Model file for the job. Use its own axes, mm. A direction names the side the tool comes from. Round coordinates to 2 decimals unless told otherwise and drop trailing zeros. Order: outer loops, then holes, each group sorted by start corner. A loop starts at its lowest first (then second) coordinate and runs counter-clockwise, first axis right, second up. Notation, with made-up numbers: M 23.25,27 L 29.25,27 A22 ccw 29.25,48 Z; hole C -28,-19.5 d5. An arc over 180 degrees is marked long. Return JSON: item names as keys, results as strings. Group by question number.
Item 1: Which spindle directions (+Z, -Z, +X, -X, +Y, -Y) get a long thin tool onto all of the face, cutting with end or side? Do faces 5 (the face through (18, -1, 12.5)), 6 (the face through (34, -2, 6)), 7 (the face through (17, -3.2, 7)), 8 (the face through (19, -2, 11.7)), 9 (the face through (4, -2, 6)). Say none if no direction does.
Item 2: Slice it at D-D on z = 5.75. Write the cut outline in (x, y).
Item 3: Pin check, flat tips, straight feed: pin 1 Ø1.3 at (x, y) = (20, -3) entering from +Z; pin 2 Ø0.5 at (y, z) = (-2.5, 7.5) entering from +X. Stop position of each tip, or through.
Item 4: Pull direction Z, two halves, no side cores. Call faces 1 (the face through (19, -3.3, 3)), 2 (the face through (19, -2, 0.2)), 3 (the face through (1.215, -0.838, 5.317)), 4 (the face through (0.948, -0.838, 7.917)): pulls with the +Z half, pulls with the -Z half, needs draft (parallel to the pull), parting line crosses it, or undercut.
Item 5: Slice it at B-B on z = 7.52. Write the cut outline in (x, y).
Item 6: Slice it at A-A on x = 1. Write the cut outline in (y, z).
Item 7: Slice it at C-C on x = 30.5. Write the cut outline in (y, z), then the cut area to 4 significant figures.
Item 8: Probe line 1 along Z through (x, y) = (1, -0.8); line 2 along X through (y, z) = (-1.1, 7.52); line 3 along Z through (x, y) = (28, -2.9). List the from-to ranges inside material, lowest first.
from build123d import *

# Parameters (mm, degrees)
SKETCH_W            = 36
SKETCH_H            = 12.5
PAD_DEPTH           = 1.7
SKETCH001_W         = 30
SKETCH001_H         = 11.5
PAD001_DEPTH        = 3.3
SKETCH002_W         = 22.38
SKETCH002_H         = 5.58
POCKET003_DEPTH     = 0.1
SKETCH003_R         = 0.4
HOLE_DEPTH          = 25
LINEARPATTERN_COUNT = 4
LINEARPATTERN_PITCH = 2.54
FILLET_R            = 0.5


with BuildPart() as part:
    # Sketch → Pad (new body)
    with BuildSketch(Plane.XZ):
        with Locations((18, 6.25)):
            Rectangle(SKETCH_W, SKETCH_H)
    extrude(amount=PAD_DEPTH)

    # Sketch001 → Pad001 (join)
    with BuildSketch(Plane.XZ):
        with Locations((19, 5.95)):
            Rectangle(SKETCH001_W, SKETCH001_H)
    extrude(amount=PAD001_DEPTH)

    # Sketch002 (on Face10 of Pad001) → Pocket003 (cut)
    with BuildSketch(Plane.XZ.offset(3.3)):
        with Locations((16.99, 7.19)):
            Rectangle(SKETCH002_W, SKETCH002_H)
    extrude(amount=-POCKET003_DEPTH, mode=Mode.SUBTRACT)

    # Sketch003 → Hole (cut)
    with BuildSketch(Plane.XZ):
        with Locations((1, 2.44)):
            Circle(SKETCH003_R)
    hole = extrude(amount=HOLE_DEPTH, mode=Mode.SUBTRACT)

    # LinearPattern: Hole ×4
    with Locations(*[(0, 0, i * LINEARPATTERN_PITCH) for i in range(1, LINEARPATTERN_COUNT)]):
        add(hole, mode=Mode.SUBTRACT)

    # Fillet
    fillet_edges = [part.edges().sort_by_distance(p)[0] for p in [
        (36, -0.85, 12.5),
        (36, -0.85, 0),
        (0, -0.85, 12.5),
        (0, -0.85, 0),
    ]]
    fillet(fillet_edges, radius=FILLET_R)


solid = part.part
Output values:
{
 "1": {"face 5": "+Z, +X, -X, +Y, -Y", "face 6": "+Z, -Z, +X, -Y", "face 7": "-Y", "face 8": "+Z, +X, -X, -Y", "face 9": "+Z, -Z, -X, -Y"},
 "2": {"outline": "M 0,-1.7 L 4,-1.7 L 4,-3.3 L 5.8,-3.3 L 5.8,-3.2 L 28.18,-3.2 L 28.18,-3.3 L 34,-3.3 L 34,-1.7 L 36,-1.7 L 36,0 L 0,0 Z"},
 "3": {"pin 1": "z = 11.7", "pin 2": "x = 34"},
 "4": {"face 1": "needs draft", "face 2": "pulls with the -Z half", "face 3": "undercut", "face 4": "undercut"},
 "5": {"outline": "M 0,-1.7 L 0.6,-1.7 L 0.6,0 L 0,0 Z; M 1.4,-1.7 L 4,-1.7 L 4,-3.3 L 5.8,-3.3 L 5.8,-3.2 L 28.18,-3.2 L 28.18,-3.3 L 34,-3.3 L 34,-1.7 L 36,-1.7 L 36,0 L 1.4,0 Z"},
 "6": {"outline": "M -1.7,0 L 0,0 L 0,2.04 L -1.7,2.04 Z; M -1.7,2.84 L 0,2.84 L 0,4.58 L -1.7,4.58 Z; M -1.7,5.38 L 0,5.38 L 0,7.12 L -1.7,7.12 Z; M -1.7,7.92 L 0,7.92 L 0,9.66 L -1.7,9.66 Z; M -1.7,10.46 L 0,10.46 L 0,12.5 L -1.7,12.5 Z"},
 "7": {"outline": "M -3.3,0.2 L -1.7,0.2 L -1.7,0 L 0,0 L 0,12.5 L -1.7,12.5 L -1.7,11.7 L -3.3,11.7 Z", "area": "39.65 mm²"},
 "8": {"line 1": "0 to 2.04, 2.84 to 4.58, 5.38 to 7.12, 7.92 to 9.66, 10.46 to 12.5", "line 2": "0 to 0.6, 1.4 to 36", "line 3": "0.2 to 11.7"}
}
